from build123d import *

# Parameters (mm, degrees)
SKETCH007_W         = 65.5
SKETCH007_H         = 65.5
SKETCH007_R         = 2.6
PAD005_DEPTH        = 5
PAD006_DEPTH        = 12
HOLE_D              = 5
HOLE_DEPTH          = 25
HOLE_CSINK_D        = 7
HOLE_CSINK_ANGLE    = 80
PAD007_DEPTH        = 12
HOLE001_D           = 5
HOLE001_DEPTH       = 25
HOLE001_CSINK_D     = 7
HOLE001_CSINK_ANGLE = 80


with BuildPart() as part:
    # Sketch007 (on Face1 of Binder) → Pad005 (new body)
    with BuildSketch(Plane.XY.offset(78)):
        Rectangle(SKETCH007_W, SKETCH007_H)
        with Locations((-20, -10)):
            Circle(SKETCH007_R, mode=Mode.SUBTRACT)
        with Locations((20, -10)):
            Circle(SKETCH007_R, mode=Mode.SUBTRACT)
        with Locations((-20, 10)):
            Circle(SKETCH007_R, mode=Mode.SUBTRACT)
        with Locations((20, 10)):
            Circle(SKETCH007_R, mode=Mode.SUBTRACT)
        Circle(SKETCH007_R, mode=Mode.SUBTRACT)
        with BuildLine():
            ThreePointArc((-10.3, -17.45), (-12.85, -20), (-10.3, -22.55))
            Line((-10.3, -22.55), (10.3, -22.55))
            ThreePointArc((10.3, -22.55), (12.85, -20), (10.3, -17.45))
            Line((-10.3, -17.45), (10.3, -17.45))
        make_face(mode=Mode.SUBTRACT)
        with BuildLine():
            ThreePointArc((10.3, 17.45), (12.85, 20), (10.3, 22.55))
            Line((10.3, 22.55), (-10.3, 22.55))
            ThreePointArc((-10.3, 22.55), (-12.85, 20), (-10.3, 17.45))
            Line((10.3, 17.45), (-10.3, 17.45))
        make_face(mode=Mode.SUBTRACT)
    extrude(amount=PAD005_DEPTH)

    # Sketch008 (on Face4 of Pad005) → Pad006 (join)
    with BuildSketch(Plane(origin=(0, 32.75, 0), x_dir=(-1, 0, 0), z_dir=(0, 1, 0))):
        Polygon((-39.678203, 87), (-54.017949, 87), (-54.017949, 82), (-41.017949, 82), (-34.089746, 78), (-32.75, 78), (-32.75, 83), align=None)
        Polygon((39.678203, 87), (54.017949, 87), (54.017949, 82), (41.017949, 82), (34.089746, 78), (32.75, 78), (32.75, 83), align=None)
    extrude(amount=-PAD006_DEPTH)

    # Hole
    with Locations(Plane(origin=(0, 0, 82), x_dir=(1, 0, 0), z_dir=(0, 0, -1))):
        with Locations((-47.517949, -26.75), (47.517949, -26.75)):
            CounterSinkHole(HOLE_D / 2, HOLE_CSINK_D / 2, depth=HOLE_DEPTH, counter_sink_angle=HOLE_CSINK_ANGLE)

    # Sketch010 (on Face3 of Hole) → Pad007 (join)
    with BuildSketch(Plane.XZ.offset(32.75)):
        Polygon((-32.75, 83), (-39.678203, 87), (-54.017949, 87), (-54.017949, 82), (-41.017949, 82), (-34.089746, 78), (-32.75, 78), align=None)
        Polygon((32.75, 78), (32.75, 83), (39.678203, 87), (54.017949, 87), (54.017949, 82), (41.017949, 82), (34.089746, 78), align=None)
    extrude(amount=-PAD007_DEPTH)

    # Hole001
    with Locations(Plane(origin=(0, 0, 82), x_dir=(1, 0, 0), z_dir=(0, 0, -1))):
        with Locations((-47.517949, 26.75), (47.517949, 26.75)):
            CounterSinkHole(HOLE001_D / 2, HOLE001_CSINK_D / 2, depth=HOLE001_DEPTH, counter_sink_angle=HOLE001_CSINK_ANGLE)


solid = part.part
Model file for the job. Use its own axes, mm. A direction names the side the tool comes from. Coordinates: 2 decimals unless noted, no trailing zeros. Write each loop counter-clockwise with the first axis right and the second up, starting at its lowest first coordinate (ties: lowest second). Pieces come first, ordered by that corner, then holes. Notation, with made-up numbers: (18.5, -11.5) -> (59.5, -11.5) arc R23 cw to (59.5, 8.5) -> close; hole circle Ø5 at (-32, 5.25). An arc over 180 degrees is marked (long way). One line per item, written item: value. Start each with the question number.
1) Slice it at D-D on z = 85.5. Write the cut outline in (x, y), then the cut area to 3 significant figures.
2) Pull direction X, two halves, no side cores. Call faces 1 (the face through (45, 24, 82)), 2 (the face through (0, 17.45, 80)), 3 (the face through (54.018, 27, 85)): +X half, -X half, draft (parallel to the pull), parting line (faces both ways), or undercut.
3) Flat gauge pins, fed straight in: pin 1 Ø6 at (x, y) = (20, 12) entering from +Z; pin 2 Ø3.5 at (x, y) = (-46, -28) entering from -Z; pin 3 Ø6 at (x, y) = (-47.52, 26.75) entering from -Z. Where does each tip first touch, or does it go through?
4) Which spindle directions (+Z, -Z, +X, -X, +Y, -Y) get a long thin tool onto all of the face, cutting with end or side? Do faces 4 (the face through (44, 20.75, 84)), 5 (the face through (36.166, -26.834, 84.972)), 6 (the face through (0, -17.45, 80)). Say none if no direction does.
5) Slice it at B-B on y = 26.75. Write the cut outline in (x, z).
6) Slice it at C-C on x = 0. Write the cut outline in (y, z).
7) Slice it at A-A on x = 20. Write the cut outline in (y, z).
8) Probe probe 1 along Y at (x, z) = (-7, 80); probe 2 along Y at (x, z) = (0, 79.5); probe 3 along Y at (x, z) = (-44.5, 85.5). List the from-to ranges inside material, lowest first.
Answers follow:
1. outline: (-54.02, -32.75) -> (-37.08, -32.75) -> (-37.08, -20.75) -> (-54.02, -20.75) -> close; (-54.02, 20.75) -> (-37.08, 20.75) -> (-37.08, 32.75) -> (-54.02, 32.75) -> close; (37.08, -32.75) -> (54.02, -32.75) -> (54.02, -20.75) -> (37.08, -20.75) -> close; (37.08, 20.75) -> (54.02, 20.75) -> (54.02, 32.75) -> (37.08, 32.75) -> close; hole circle Ø5 at (-47.52, -26.75); hole circle Ø5 at (-47.52, 26.75); hole circle Ø5 at (47.52, -26.75); hole circle Ø5 at (47.52, 26.75)
1. area: 734 mm2
2. face 1: draft
2. face 2: undercut
2. face 3: +X half
3. pin 1: z = 83
3. pin 2: z = 82
3. pin 3: z = 82.59
4. face 4: +Z, -Z, +X
4. face 5: +Z, +Y, -Y
4. face 6: +Z, -Z
5. outline: (-54.02, 82) -> (-51.02, 82) -> (-50.02, 83.19) -> (-50.02, 87) -> (-54.02, 87) -> close; (-45.02, 83.19) -> (-44.02, 82) -> (-41.02, 82) -> (-34.09, 78) -> (34.09, 78) -> (41.02, 82) -> (44.02, 82) -> (45.02, 83.19) -> (45.02, 87) -> (39.68, 87) -> (32.75, 83) -> (-32.75, 83) -> (-39.68, 87) -> (-45.02, 87) -> close; (50.02, 83.19) -> (51.02, 82) -> (54.02, 82) -> (54.02, 87) -> (50.02, 87) -> close
6. outline: (-32.75, 78) -> (-22.55, 78) -> (-22.55, 83) -> (-32.75, 83) -> close; (-17.45, 78) -> (-2.6, 78) -> (-2.6, 83) -> (-17.45, 83) -> close; (2.6, 78) -> (17.45, 78) -> (17.45, 83) -> (2.6, 83) -> close; (22.55, 78) -> (32.75, 78) -> (32.75, 83) -> (22.55, 83) -> close
7. outline: (-32.75, 78) -> (-12.6, 78) -> (-12.6, 83) -> (-32.75, 83) -> close; (-7.4, 78) -> (7.4, 78) -> (7.4, 83) -> (-7.4, 83) -> close; (12.6, 78) -> (32.75, 78) -> (32.75, 83) -> (12.6, 83) -> close
8. probe 1: -32.75 to -22.55, -17.45 to 17.45, 22.55 to 32.75
8. probe 2: -32.75 to -22.55, -17.45 to -2.6, 2.6 to 17.45, 22.55 to 32.75
8. probe 3: -32.75 to -20.75, 20.75 to 32.75
